The model under review builds one solid part; all positions refer to its coordinate system, in mm. Coordinates: 2 decimals unless noted, no trailing zeros. Order: outer loops, then holes, each group sorted by start corner. A loop starts at its lowest first (then second) coordinate and runs counter-clockwise, first axis right, second up. Notation, with made-up numbers: (44, -2.5) - (81, -2.5) arc R32 cw to (81, 34.5) - close; hole circle Ø11 at (75.5, -35). An arc over 180 degrees is marked (long way). Answer in a Markdown table with one row per item.
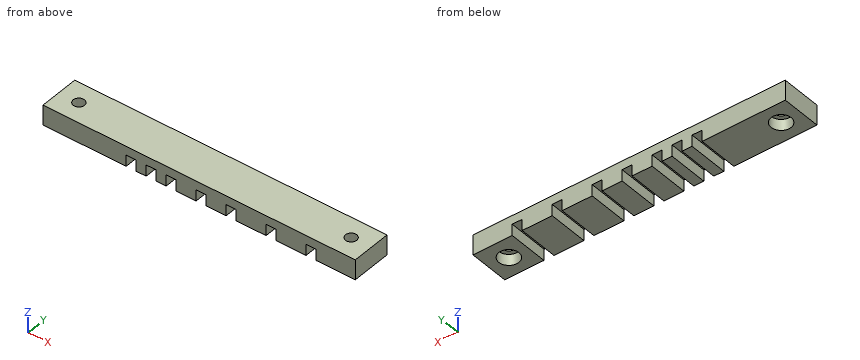
```python
from build123d import *

# Parameters (mm, degrees)
SKETCH2_W           = 125
SKETCH2_H           = 16
BOSS_EXTRUDE1_DEPTH = 8
SKETCH3_W           = 4
SKETCH3_H           = 6.863597229
SKETCH3_H_2         = 10.419332053
CUT_EXTRUDE1_DEPTH  = 17
SKETCH4_R           = 4
CUT_EXTRUDE2_DEPTH  = 4.4
SKETCH5_R           = 2.25
CUT_EXTRUDE3_DEPTH  = 4.6


with BuildPart() as part:
    # Sketch2 → Boss-Extrude1 (new body)
    with BuildSketch(Plane.XY):
        with Locations((3.707075963, 6.242976067)):
            Rectangle(SKETCH2_W, SKETCH2_H)
    extrude(amount=BOSS_EXTRUDE1_DEPTH)

    # Sketch3 → Cut-Extrude1 (cut, through all)
    with BuildSketch(Plane(origin=(0, 14.242976067, 0), x_dir=(1, 0, 0), z_dir=(0, 1, 0))):
        with Locations((48.507075963, -1.068201385)):
            Rectangle(SKETCH3_W, SKETCH3_H)
        with Locations((32.507075963, 0.709666027)):
            Rectangle(SKETCH3_W, SKETCH3_H_2)
        with Locations((16.507075963, 0.709666027)):
            Rectangle(SKETCH3_W, SKETCH3_H_2)
        with Locations((4.507075963, 0.709666027)):
            Rectangle(SKETCH3_W, SKETCH3_H_2)
        with Locations((-7.492924037, 0.709666027)):
            Rectangle(SKETCH3_W, SKETCH3_H_2)
        with Locations((-15.492924037, 0.709666027)):
            Rectangle(SKETCH3_W, SKETCH3_H_2)
        with Locations((-23.492924037, 0.709666027)):
            Rectangle(SKETCH3_W, SKETCH3_H_2)
    extrude(amount=-CUT_EXTRUDE1_DEPTH, mode=Mode.SUBTRACT)

    # Sketch4 → Cut-Extrude2 (cut)
    with BuildSketch(Plane(origin=(0, 0, 0), x_dir=(-1, 0, 0), z_dir=(0, 0, -1))):
        with Locations((50.792924037, 6.242976067)):
            Circle(SKETCH4_R)
        with Locations((-58.207075963, 6.242976067)):
            Circle(SKETCH4_R)
    extrude(amount=-CUT_EXTRUDE2_DEPTH, mode=Mode.SUBTRACT)

    # Sketch5 → Cut-Extrude3 (cut, through all)
    with BuildSketch(Plane(origin=(0, 0, 4.4), x_dir=(-1, 0, 0), z_dir=(0, 0, -1))):
        with Locations((50.792924037, 6.242976067)):
            Circle(SKETCH5_R)
        with Locations((-58.207075963, 6.242976067)):
            Circle(SKETCH5_R)
    extrude(amount=-CUT_EXTRUDE3_DEPTH, mode=Mode.SUBTRACT)


solid = part.part
```
Item 1: Clearance check with flat-ended pins moving along their axes: pin 1 Ø2.5 at (x, y) = (-49.5, 4.5) entering from -Z; pin 2 Ø1.2 at (x, y) = (32, 4.5) entering from -Z. State where each tip first meets the part, or that it passes through.
Check values:
| item | result |
|---|---|
| pin 1 | z = 4.4 |
| pin 2 | z = 4.5 |
Item 2: We need section C-C, the plane x = 57. Write out the cut boundary in (y, z), then the cut area to 3 significant figures.
Check values:
| item | result |
|---|---|
| outline | (-1.76, 0) - (2.43, 0) - (2.43, 4.4) - (4.34, 4.4) - (4.34, 8) - (-1.76, 8) - close; (8.14, 4.4) - (10.06, 4.4) - (10.06, 0) - (14.24, 0) - (14.24, 8) - (8.14, 8) - close |
| area | 80.8 mm^2 |
Item 3: To check wall thickness, follow line 1 (X direction, y = 6, z = 6); line 2 (X direction, y = 7, z = 5.25); line 3 (Y direction, x = -50.5, z = 6). State the ranges of each line that lie inside material, in increasing order. Write a range as from..to.
Check values:
| item | result |
|---|---|
| line 1 | -58.79..-53.03, -48.56..55.97, 60.44..66.21 |
| line 2 | -58.79..-52.91, -48.67..56.09, 60.33..66.21 |
| line 3 | -1.76..4.01, 8.47..14.24 |
Item 4: We need section A-A, the plane z = 2.75. State how many separate pieces and enclosed holes the cut face has, then the cut area to 3 significant figures.
Check values:
| item | result |
|---|---|
| separate pieces | 8 |
| enclosed holes | 2 |
| area | 1,450 mm^2 |
